Input: part model. Units: mm. Frame: model coordinates. Face numbers are marked on the shaded views. A direction names the side the tool comes from. Round coordinates to 2 decimals unless told otherwise and drop trailing zeros. Order: outer loops, then holes, each group sorted by start corner. A loop starts at its lowest first (then second) coordinate and runs counter-clockwise, first axis right, second up.
Item 1: Cut plane D-D on y = 245. Output: boundary loops of the cut face in (x, z).
Item 2: Cut plane A-A on x = 110. Output: boundary loops of the cut face in (y, z), then the cut area to 3 significant figures.
Item 3: Line query: L1, parallel to Y at x = 101.5, z = -23.84; L2, parallel to X at y = 245, z = -25.5; L3, parallel to Y at x = 190, z = -26.3. Output: solid intervals per line, ascending.
Item 4: Cut plane C-C on x = 70. Output: boundary loops of the cut face in (y, z).
Item 5: First-contact query: pin 1 (2 mm diameter, centred on x = 64, z = -25.5, fed in from +Y); pin 2 (3 mm diameter, centred on y = 233.5, z = -22, fed in from -X); pin 3 (3 mm diameter, centred on y = 274.5, z = -23, fed in from +X); pin 4 (1.9 mm diameter, centred on y = 274, z = -24.5, fed in from -X). Flat tips, straight axial feed; report the tip coordinate or a pass-through.
Item 6: Reachability of the marked faces 1 and 2 from +Z, -Z, +X, -X, +Y, -Y: full face, straight path, thin tool, end or side. Return the list, or none.
Item 7: Cut plane B-B on y = 257. Output: boundary loops of the cut face in (x, z).
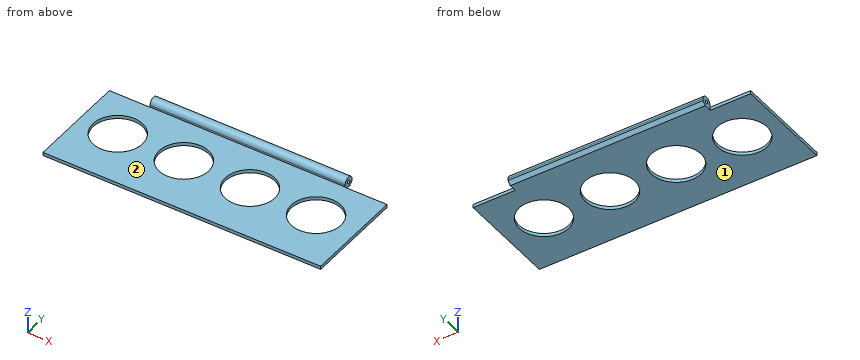
```python
from build123d import *

# Parameters (mm, degrees)
SKETCH137_R      = 15
EXTRUDE127_DEPTH = 4
SKETCH078_W      = 25.5
SKETCH078_H      = 8
EXTRUDE070_DEPTH = 7
SKETCH075_R      = 1.16
EXTRUDE067_DEPTH = 168


with BuildPart() as extrude127:
    # Sketch137 → Extrude127 (new body)
    with BuildSketch(Plane(origin=(0, 0, -28), x_dir=(1, 0, 0), z_dir=(0, 0, -1))):
        with Locations((150, -245)):
            Circle(SKETCH137_R)
        with Locations((190, -245)):
            Circle(SKETCH137_R)
        with Locations((70, -245)):
            Circle(SKETCH137_R)
        with Locations((110, -245)):
            Circle(SKETCH137_R)
    extrude(amount=-EXTRUDE127_DEPTH)


with BuildPart() as compound026:
    # Sketch078 → Extrude070 (new body)
    with BuildSketch(Plane(origin=(0, 279, 0), x_dir=(-1, 0, 0), z_dir=(0, 1, 0))):
        with Locations((-202.25, -24)):
            Rectangle(SKETCH078_W, SKETCH078_H)
        with Locations((-58.75, -24)):
            Rectangle(SKETCH078_W, SKETCH078_H)
    extrude(amount=-EXTRUDE070_DEPTH)

    # Compound026: union Extrude127
    add(extrude127.part)


with BuildPart() as battery_lid:
    # Sketch075 → Extrude067 (new body)
    with BuildSketch(Plane.YZ.offset(47)):
        with BuildLine():
            Line((272.18, -25), (211.5, -25))
            Line((211.5, -25), (211.5, -27))
            Line((211.5, -27), (276.5, -27))
            Line((278.5, -25), (276.5, -27))
            Line((278.5, -25), (278.5, -23.84))
            ThreePointArc((278.5, -23.84), (275.34, -20.68), (272.18, -23.84))
            Line((272.18, -23.84), (272.18, -25))
        make_face()
        with Locations((275.34, -23.84)):
            Circle(SKETCH075_R, mode=Mode.SUBTRACT)
    extrude(amount=EXTRUDE067_DEPTH)

    # Cut014: cut Compound026
    add(compound026.part, mode=Mode.SUBTRACT)


solid = battery_lid.part
```
From the geometry:
1. outline: (47, -27) - (55, -27) - (55, -25) - (47, -25) - close; (85, -27) - (95, -27) - (95, -25) - (85, -25) - close; (125, -27) - (135, -27) - (135, -25) - (125, -25) - close; (165, -27) - (175, -27) - (175, -25) - (165, -25) - close; (205, -27) - (215, -27) - (215, -25) - (205, -25) - close
2. outline: (211.5, -27) - (230, -27) - (230, -25) - (211.5, -25) - close; (260, -27) - (276.5, -27) - (278.5, -25) - (278.5, -23.84) arc R3.16 ccw to (272.18, -23.84) - (272.18, -25) - (260, -25) - close; hole circle Ø2.32 at (275.34, -23.84)
2. area: 90.8 mm2
3. L1: y = 272.18 to 274.18, 276.5 to 278.5
3. L2: x = 47 to 55, 85 to 95, 125 to 135, 165 to 175, 205 to 215
3. L3: y = 211.5 to 230, 260 to 272
4. outline: (211.5, -27) - (230, -27) - (230, -25) - (211.5, -25) - close; (260, -27) - (272, -27) - (272, -25) - (260, -25) - close
5. pin 1: stops at y = 272
5. pin 2: passes through
5. pin 3: stops at x = 189.5
5. pin 4: stops at x = 71.5
6. face 1: -Z, +X, -X, +Y, -Y
6. face 2: +Z, +X, -X, -Y
7. outline: (47, -27) - (61, -27) - (61, -25) - (47, -25) - close; (79, -27) - (101, -27) - (101, -25) - (79, -25) - close; (119, -27) - (141, -27) - (141, -25) - (119, -25) - close; (159, -27) - (181, -27) - (181, -25) - (159, -25) - close; (199, -27) - (215, -27) - (215, -25) - (199, -25) - close
